Geometry: final body of the model. Coordinates: model frame, mm. A direction names the side the tool comes from. Round coordinates to 2 decimals unless told otherwise and drop trailing zeros. Write each loop counter-clockwise with the first axis right and the second up, starting at its lowest first coordinate (ties: lowest second). Pieces come first, ordered by that corner, then holes. Notation, with made-up numbers: M 18.25,44.25 L 60.25,44.25 A29 cw 60.25,71.25 Z; hole C 16.5,-15 d1. An arc over 180 degrees is marked long. Use one line per item in the form item = value. Start each with the question number.
Item 1: Reachability of faces 1 (the cylindrical face through (-7.13, 49.67, 3.06)), 2 (the flat face through (12, -53.5, 3)), 3 (the flat face through (92.1, -111, 3)) from +Z, -Z, +X, -X, +Y, -Y: full face, straight path, thin tool, end or side. Return the list, or none.
Item 2: Section query D-D (y = -3.5). Return loops of the section in (x, z), and give its area (3 significant figures).
Item 3: Section query B-B (x = -4.85). Return loops of the section in (y, z).
Item 4: Section query A-A (y = -50.4). Return loops of the section in (x, z), and give its area (3 significant figures).
Item 5: Pin query (flat end, axial travel): pin 1 Ø1.5 at (y, z) = (-98.5, 1) entering from -X; pin 2 Ø3 at (y, z) = (16.5, 1.5) entering from +X; pin 3 Ø1.6 at (x, z) = (-28, 4.5) entering from +Y. Return the tip coordinate at first contact, or that it passes through.
Item 6: Pull-direction query (Y, two-part tool) for faces 4 (the flat face through (61, -88, 3)), 5 (the flat face through (-33.65, -98, 3)), 6 (the cylindrical face through (39.442, 52.503, 3.057)), 7 (the flat face through (-18, -113, 3)); classes: pulls with the +Y half, pulls with the -Y half, needs draft (parallel to the pull), parting line crosses it, or undercut.
Item 7: Section query C-C (y = -71). Return loops of the section in (x, z), and give its area (3 significant figures).
Item 8: Ray query, probe 1 along Y at (x, z) = (-48, 3.5); probe 2 along Y at (x, z) = (-5.5, 1.75); probe 3 along X at (y, z) = (-2, 5.25). Return the intervals inside material, ascending.
from build123d import *

# Parameters (mm, degrees)
SKETCH1_R           = 4
SKETCH1_R_2         = 3
SKETCH1_R_3         = 9
BOSS_EXTRUDE1_DEPTH = 6.2
CUT_EXTRUDE1_REACH  = 156.506
SKETCH2_R           = 1.5
CUT_EXTRUDE2_REACH  = 156.506
CUT_EXTRUDE3_REACH  = 156.506
SKETCH5_R           = 3
SKETCH5_W           = 8
SKETCH5_H           = 6.2


with BuildPart() as part:
    # Sketch1 → Boss-Extrude1 (new body)
    with BuildSketch(Plane.XY):
        with BuildLine():
            Line((-57.678304402, -8.5), (-47, -26.5))
            Line((-47, -26.5), (-33.65, -83.5))
            Line((-33.65, -83.5), (-33.65, -113))
            Line((-33.65, -113), (-15.15, -113))
            Line((-15.15, -113), (-15.15, -119))
            Line((-15.15, -119), (79.85, -119))
            Line((79.85, -119), (79.85, -113))
            Line((79.85, -113), (98.35, -113))
            Line((98.35, -113), (98.35, -28.5))
            ThreePointArc((98.35, -28.5), (73.847295802, 13.224376921), (42.748141943, 50.293889619))
            ThreePointArc((42.748141943, 50.293889619), (39.389057397, 52.524667098), (35.422008956, 53.247400666))
            ThreePointArc((35.422008956, 53.247400666), (-7.727235636, 49.583712908), (-50.093777716, 40.619560464))
            ThreePointArc((-50.093777716, 40.619560464), (-56.473591535, 35.874651698), (-58, 28.071686829))
            Line((-58, 28.071686829), (-54, 5.071686829))
            ThreePointArc((-54, 5.071686829), (-58.708572703, -0.936463864), (-57.678304402, -8.5))
        make_face()
        with Locations(Location((-47.15, 30, 0), (0, 0, 180))):
            Circle(SKETCH1_R, mode=Mode.SUBTRACT)
        with Locations(Location((27.65, 40.9, 0), (0, 0, 180))):
            Circle(SKETCH1_R_2, mode=Mode.SUBTRACT)
        with Locations(Location((-4.85, -80.4, 0), (0, 0, 180))):
            Circle(SKETCH1_R_2, mode=Mode.SUBTRACT)
        with Locations(Location((-49.25, -3.5, 0), (0, 0, 180))):
            Circle(SKETCH1_R_2, mode=Mode.SUBTRACT)
        with Locations(Location((72, -36, 0), (0, 0, 180))):
            Circle(SKETCH1_R_2, mode=Mode.SUBTRACT)
        with Locations(Location((0, 0, 0), (0, 0, 180))):
            Circle(SKETCH1_R_3, mode=Mode.SUBTRACT)
        with BuildLine():
            Line((82.35, -64), (82.35, -82))
            ThreePointArc((82.35, -82), (80.592640687, -86.242640687), (76.35, -88))
            Line((76.35, -88), (45.35, -88))
            ThreePointArc((45.35, -88), (39.556365472, -83.560063768), (42.337186896, -76.81126632))
            Line((42.337186896, -76.81126632), (73.337186896, -58.81126632))
            ThreePointArc((73.337186896, -58.81126632), (79.343586593, -58.800150068), (82.35, -64))
        make_face(mode=Mode.SUBTRACT)
    extrude(amount=BOSS_EXTRUDE1_DEPTH)

    # Sketch2 → Cut-Extrude1 (cut, up to next)
    with BuildSketch(Plane.XY.offset(6.2), mode=Mode.PRIVATE) as cut_extrude1_sk1:
        with Locations((19.348702159, -20.792251556)):
            Circle(SKETCH2_R)
    cut_extrude1_tool1 = extrude(cut_extrude1_sk1.sketch, amount=-CUT_EXTRUDE1_REACH, mode=Mode.PRIVATE) & part.part
    # Sketch2 → Cut-Extrude1 (cut, up to next)
    with BuildSketch(Plane.XY.offset(6.2), mode=Mode.PRIVATE) as cut_extrude1_sk2:
        with Locations((-11.192862241, -26.103827973)):
            Circle(SKETCH2_R)
    cut_extrude1_tool2 = extrude(cut_extrude1_sk2.sketch, amount=-CUT_EXTRUDE1_REACH, mode=Mode.PRIVATE) & part.part
    # Sketch2 → Cut-Extrude1 (cut, up to next)
    with BuildSketch(Plane.XY.offset(6.2), mode=Mode.PRIVATE) as cut_extrude1_sk3:
        with Locations((-16.504438658, 4.437736426)):
            Circle(SKETCH2_R)
    cut_extrude1_tool3 = extrude(cut_extrude1_sk3.sketch, amount=-CUT_EXTRUDE1_REACH, mode=Mode.PRIVATE) & part.part
    # Sketch2 → Cut-Extrude1 (cut, up to next)
    with BuildSketch(Plane.XY.offset(6.2), mode=Mode.PRIVATE) as cut_extrude1_sk4:
        with Locations((14.037125741, 9.749312843)):
            Circle(SKETCH2_R)
    cut_extrude1_tool4 = extrude(cut_extrude1_sk4.sketch, amount=-CUT_EXTRUDE1_REACH, mode=Mode.PRIVATE) & part.part
    add(cut_extrude1_tool1.solids().sort_by_distance((19.348702, -20.792252, 6.2))[0], mode=Mode.SUBTRACT)
    add(cut_extrude1_tool2.solids().sort_by_distance((-11.192862, -26.103828, 6.2))[0], mode=Mode.SUBTRACT)
    add(cut_extrude1_tool3.solids().sort_by_distance((-16.504439, 4.437736, 6.2))[0], mode=Mode.SUBTRACT)
    add(cut_extrude1_tool4.solids().sort_by_distance((14.037126, 9.749313, 6.2))[0], mode=Mode.SUBTRACT)

    # Sketch3 → Cut-Extrude2 (cut, up to next)
    with BuildSketch(Plane.XY.offset(6.2), mode=Mode.PRIVATE) as cut_extrude2_sk1:
        Polygon((-29.4, -103), (-19.4, -103), (-19.4, -108), (-21.4, -108), (-21.4, -113), (-27.4, -113), (-27.4, -108), (-29.4, -108), align=None)
    cut_extrude2_tool1 = extrude(cut_extrude2_sk1.sketch, amount=-CUT_EXTRUDE2_REACH, mode=Mode.PRIVATE) & part.part
    # Sketch3 → Cut-Extrude2 (cut, up to next)
    with BuildSketch(Plane.XY.offset(6.2), mode=Mode.PRIVATE) as cut_extrude2_sk2:
        Polygon((86.1, -108), (86.1, -113), (92.1, -113), (92.1, -108), (94.1, -108), (94.1, -103), (84.1, -103), (84.1, -108), align=None)
    cut_extrude2_tool2 = extrude(cut_extrude2_sk2.sketch, amount=-CUT_EXTRUDE2_REACH, mode=Mode.PRIVATE) & part.part
    add(cut_extrude2_tool1.solids().sort_by_distance((-24.4, -107.375, 6.2))[0], mode=Mode.SUBTRACT)
    add(cut_extrude2_tool2.solids().sort_by_distance((89.1, -107.375, 6.2))[0], mode=Mode.SUBTRACT)

    # Sketch5 → Cut-Extrude3 (cut, up to next)
    with BuildSketch(Plane.XY.offset(6.2), mode=Mode.PRIVATE) as cut_extrude3_sk1:
        with Locations((24.05, -50.4)):
            Circle(SKETCH5_R)
    cut_extrude3_tool1 = extrude(cut_extrude3_sk1.sketch, amount=-CUT_EXTRUDE3_REACH, mode=Mode.PRIVATE) & part.part
    # Sketch5 → Cut-Extrude3 (cut, up to next)
    with BuildSketch(Plane.XY.offset(6.2), mode=Mode.PRIVATE) as cut_extrude3_sk2:
        with Locations((36.05, -50.4)):
            Rectangle(SKETCH5_W, SKETCH5_H)
    cut_extrude3_tool2 = extrude(cut_extrude3_sk2.sketch, amount=-CUT_EXTRUDE3_REACH, mode=Mode.PRIVATE) & part.part
    # Sketch5 → Cut-Extrude3 (cut, up to next)
    with BuildSketch(Plane.XY.offset(6.2), mode=Mode.PRIVATE) as cut_extrude3_sk3:
        with Locations((12.05, -50.4)):
            Rectangle(SKETCH5_W, SKETCH5_H)
    cut_extrude3_tool3 = extrude(cut_extrude3_sk3.sketch, amount=-CUT_EXTRUDE3_REACH, mode=Mode.PRIVATE) & part.part
    add(cut_extrude3_tool1.solids().sort_by_distance((24.05, -50.4, 6.2))[0], mode=Mode.SUBTRACT)
    add(cut_extrude3_tool2.solids().sort_by_distance((36.05, -50.4, 6.2))[0], mode=Mode.SUBTRACT)
    add(cut_extrude3_tool3.solids().sort_by_distance((12.05, -50.4, 6.2))[0], mode=Mode.SUBTRACT)


solid = part.part
Working result:
q1.face_1 = +Z, -Z, -X, +Y
q1.face_2 = +Z, -Z
q1.face_3 = +Z, -Z, -Y
q2.outline = M -59.05,0 L -52.25,0 L -52.25,6.2 L -59.05,6.2 Z; M -46.25,0 L -8.29,0 L -8.29,6.2 L -46.25,6.2 Z; M 8.29,0 L 84.81,0 L 84.81,6.2 L 8.29,6.2 Z
q2.area = 752 mm²
q3.outline = M -119,0 L -83.4,0 L -83.4,6.2 L -119,6.2 Z; M -77.4,0 L -7.58,0 L -7.58,6.2 L -77.4,6.2 Z; M 7.58,0 L 50,0 L 50,6.2 L 7.58,6.2 Z
q4.outline = M -41.4,0 L 8.05,0 L 8.05,6.2 L -41.4,6.2 Z; M 16.05,0 L 21.05,0 L 21.05,6.2 L 16.05,6.2 Z; M 27.05,0 L 32.05,0 L 32.05,6.2 L 27.05,6.2 Z; M 40.05,0 L 98.35,0 L 98.35,6.2 L 40.05,6.2 Z
q4.area = 730 mm²
q5.pin_1 = -33.65
q5.pin_2 = 72.58
q5.pin_3 = 46.14
q6.face_4 = undercut
q6.face_5 = needs draft
q6.face_6 = pulls with the +Y half
q6.face_7 = pulls with the -Y half
q7.outline = M -36.58,0 L 52.35,0 L 52.35,6.2 L -36.58,6.2 Z; M 82.35,0 L 98.35,0 L 98.35,6.2 L 82.35,6.2 Z
q7.area = 651 mm²
q8.probe_1 = -24.81 to -6.23, -0.77 to 26.09, 33.91 to 41.19
q8.probe_2 = -119 to -83.33, -77.47 to -7.12, 7.12 to 49.91
q8.probe_3 = -58.93 to -51.85, -46.65 to -8.77, 8.77 to 83.89
